from build123d import *

# Parameters (mm, degrees)
F2_W      = 74
F2_H      = 8
F2_R      = 3
F5_DEPTH  = 5
F0_R      = 1.7
F6_DEPTH  = 12.5
F3_R      = 2.05
F7_DEPTH  = 2
F8_DEPTH  = 2
F10_DEPTH = 2.4
F11_R     = 3.99999
F4_R      = 1.2
F12_DEPTH = 5.001


# Not quite as in the source:
# - a fillet or chamfer is up to 0.001 mm smaller than in the source, because OpenCascade refuses the exact size


with BuildPart() as f5:
    # F2 (on face) → F5 (new body)
    with BuildSketch(Plane.XY):
        with Locations((0, 38)):
            Rectangle(F2_W, F2_H)
        with Locations((-33, 38)):
            Circle(F2_R, mode=Mode.SUBTRACT)
        Polygon((1.1402667816, 36.025), (0, 36.025), (-1.1402667816, 36.025), (-2.2805335633, 38), (-1.1402667816, 39.975), (0, 39.975), (1.1402667816, 39.975), (2.2805335633, 38), align=None, mode=Mode.SUBTRACT)
        with Locations((33, 38)):
            Circle(F2_R, mode=Mode.SUBTRACT)
        Polygon((-1.1402667816, 36.025), (0, 36.025), (1.1402667816, 36.025), (2.2805335633, 38), (1.1402667816, 39.975), (0, 39.975), (-1.1402667816, 39.975), (-2.2805335633, 38), align=None)
        with Locations((-33, 38)):
            Circle(F2_R)
        with Locations((33, 38)):
            Circle(F2_R)
    extrude(amount=F5_DEPTH)

    # F0 (on Top) → F6 (cut, symmetric)
    with BuildSketch(Plane.XY):
        with Locations((-33, 38)):
            Circle(F0_R)
        with Locations((33, 38)):
            Circle(F0_R)
        with Locations((-33, -38)):
            Circle(F0_R)
        with Locations((33, -38)):
            Circle(F0_R)
    extrude(amount=F6_DEPTH, both=True, mode=Mode.SUBTRACT)

    # F3 (on face) → F7 (cut)
    with BuildSketch(Plane.XY):
        with Locations((-7.225, 38)):
            Circle(F3_R)
        with Locations((7.225, 38)):
            Circle(F3_R)
    extrude(amount=F7_DEPTH, mode=Mode.SUBTRACT)

    # F2 (on face) → F8 (cut)
    with BuildSketch(Plane.XY):
        Polygon((-1.1402667816, 36.025), (0, 36.025), (1.1402667816, 36.025), (2.2805335633, 38), (1.1402667816, 39.975), (0, 39.975), (-1.1402667816, 39.975), (-2.2805335633, 38), align=None)
    extrude(amount=F8_DEPTH, mode=Mode.SUBTRACT)

    # F9 (on face) → F10 (cut)
    with BuildSketch(Plane.XY.offset(5)):
        Polygon((-34.5732794835, 35.275), (-33, 35.275), (-31.4267205165, 35.275), (-29.8534410329, 38), (-31.4267205165, 40.725), (-33, 40.725), (-34.5732794835, 40.725), (-36.1465589671, 38), align=None)
        Polygon((29.8534410329, 38), (31.4267205165, 35.275), (33, 35.275), (34.5732794835, 35.275), (36.1465589671, 38), (34.5732794835, 40.725), (33, 40.725), (31.4267205165, 40.725), align=None)
    extrude(amount=-F10_DEPTH, mode=Mode.SUBTRACT)

    # F11 (radius 4 in the source; OpenCascade refuses exactly that, so slightly less here)
    f11_edges = [f5.edges().sort_by_distance(p)[0] for p in [
        (-37, 42, 2.5),
        (-37, 34, 2.5),
        (37, 42, 2.5),
        (37, 34, 2.5),
    ]]
    fillet(f11_edges, radius=F11_R)

    # F4 (on face) → F12 (cut, through all)
    with BuildSketch(Plane.XY):
        with Locations((-7.225, 38)):
            Circle(F4_R)
        with Locations((0, 38)):
            Circle(F4_R)
        with Locations((7.225, 38)):
            Circle(F4_R)
    extrude(amount=F12_DEPTH, mode=Mode.SUBTRACT)


solid = f5.part
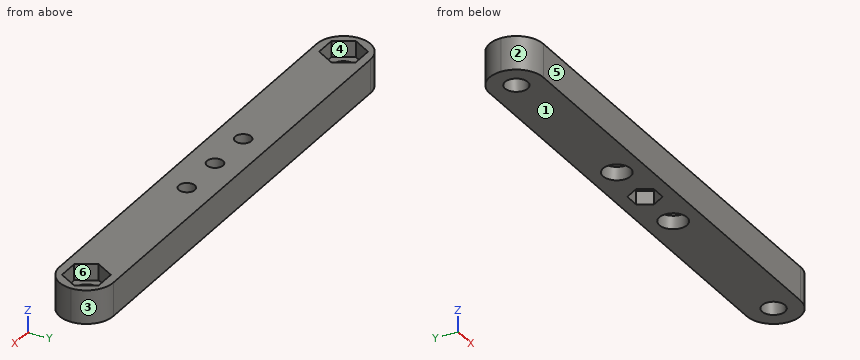
Verification items for the finished model (mm, model axes). Face numbers are marked on the shaded views. A direction names the side the tool comes from. Give positions to 0.01 mm unless a question says otherwise; leave off trailing zeros. Loops run counter-clockwise (first coordinate to the right, second up) from the corner with the lowest first, then second, coordinate; pieces in that order, holes last. Notation, with made-up numbers: (10.25, 61) - (69.25, 61) arc R29 cw to (69.25, 97) - close; hole circle Ø1 at (27.5, -26.5). An arc over 180 degrees is marked (long way). Write each question's results on one line, items separated by ' | '.
1) Sectioned sample at A-A on z = 1.05. Count the separate pieces of the cut face and the enclosed holes in it, plus the area to 3 significant figures.
Solution:
separate pieces: 1 | enclosed holes: 5 | area: 520 mm2
2) Tool access check on the marked faces 5 and 6. Record the directions out of +Z, -Z, +X, -X, +Y, -Y that give a thin tool (end or side, any length) a straight path to the whole face; none if there is none.
Solution:
face 5: +Z, -Z, +X, -X, -Y | face 6: +Z
3) Sectioned sample at B-B on x = 0. Record the boundary of the cut face in (y, z) (3 decimals).
Solution:
outline: (34, 0) - (36.025, 0) - (36.025, 2) - (36.8, 2) - (36.8, 5) - (34, 5) - close; (39.2, 2) - (39.975, 2) - (39.975, 0) - (42, 0) - (42, 5) - (39.2, 5) - close
4) Material ranges on L1, parallel to X at y = 38, z = 3.5 (3 decimals); L2, parallel to Y at x = 0, z = 3.25; L3, parallel to Y at x = 1, z = 1.25 (3 decimals), recorded low to high. Write a range as from..to.
Solution:
L1: -37..-36.147, -29.853..-8.425, -6.025..-1.2, 1.2..6.025, 8.425..29.853, 36.147..37 | L2: 34..36.8, 39.2..42 | L3: 34..36.025, 39.975..42
5) Mould release check, pull along X, two halves, no side actions. Record for the marked faces 1, 2, 3 and 4: pulls with the +X half, pulls with the -X half, needs draft (parallel to the pull), parting line crosses it, or undercut.
Solution:
face 1: needs draft | face 2: pulls with the -X half | face 3: pulls with the +X half | face 4: undercut
6) Depth check by flat-ended pin: P1, Ø1.2, axis at x = 8, y = 38.5, coming from the -Z side; P2, Ø1.5, axis at y = 39, z = 4, coming from the +X side. Enter the tip coordinate at first touch or a pass-through.
Solution:
P1: z = 2 | P2: x = 36.99
